The figure shows three views and two pictorial views of one solid part (mm, origin at its lowest corner). Answer the questions. A direction names the side the tool comes from. Coordinates: 2 decimals unless noted, no trailing zeros. Loops run counter-clockwise (first coordinate to the right, second up) from the corner with the lowest first, then second, coordinate; pieces in that order, holes last.
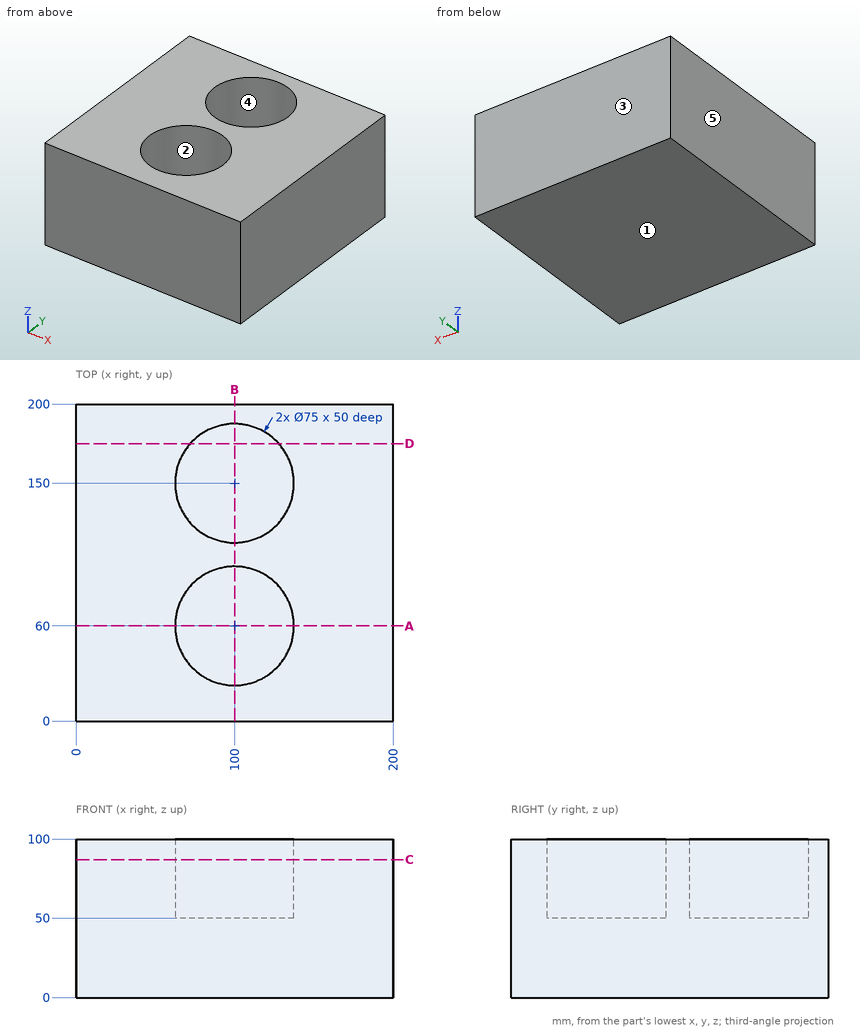
1. A cutting plane is placed at D-D, the plane y = 175. Give the vertices of the cut face in (x, z).
2. For the marked faces 1 and 2, determine the directions among +Z, -Z, +X, -X, +Y, -Y from which every point of the face is accessible in a straight line to the end or side of a thin tool.
3. A cutting plane is placed at C-C, the plane z = 87. Give the vertices of the cut face in (x, y), then the cut area to 3 significant figures.
4. A cutting plane is placed at A-A, the plane y = 60. Give the vertices of the cut face in (x, z), then the cut area to 4 significant figures.
5. Straight lines are drawn through the part: probe 1 along Y at (x, z) = (100, 80); probe 2 along Y at (x, z) = (133.5, 50.5); probe 3 along Z at (x, y) = (93, 68.5). For each, find the intervals that lie inside material, in ascending order.
6. A cutting plane is placed at B-B, the plane x = 100. Give the vertices of the cut face in (y, z).
7. Determine the mould class of the marked faces 3, 4 and 5 for opening direction Y: released by +Y, released by -Y, zero draft, split by the parting line, or undercut.
Answers below:
1. outline: (0, 0) - (200, 0) - (200, 100) - (127.95, 100) - (127.95, 50) - (72.05, 50) - (72.05, 100) - (0, 100) - close
2. face 1: -Z, +X, -X, +Y, -Y
2. face 2: +Z
3. outline: (0, 0) - (200, 0) - (200, 200) - (0, 200) - close; hole circle Ø75 at (100, 60); hole circle Ø75 at (100, 150)
3. area: 31,200 mm2
4. outline: (0, 0) - (200, 0) - (200, 100) - (137.5, 100) - (137.5, 50) - (62.5, 50) - (62.5, 100) - (0, 100) - close
4. area: 16,250 mm2
5. probe 1: y = 0 to 22.5, 97.5 to 112.5, 187.5 to 200
5. probe 2: y = 0 to 43.15, 76.85 to 133.15, 166.85 to 200
5. probe 3: z = 0 to 50
6. outline: (0, 0) - (200, 0) - (200, 100) - (187.5, 100) - (187.5, 50) - (112.5, 50) - (112.5, 100) - (97.5, 100) - (97.5, 50) - (22.5, 50) - (22.5, 100) - (0, 100) - close
7. face 3: released by +Y
7. face 4: undercut
7. face 5: zero draft
